The model under review builds one solid part; all positions refer to its coordinate system, in mm. Coordinates: 2 decimals unless noted, no trailing zeros. Order: outer loops, then holes, each group sorted by start corner. A loop starts at its lowest first (then second) coordinate and runs counter-clockwise, first axis right, second up.
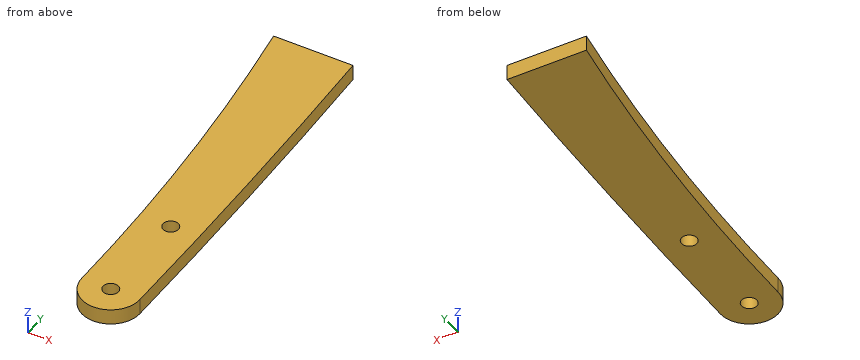
```python
from build123d import *

# Parameters (mm, degrees)
LEG_DEPTH       = 3.048
SKETCH4_R       = 1.524
FEETHOLES_DEPTH = 3.048


with BuildPart() as part:
    # Sketch3 → Leg (new body)
    with BuildSketch(Plane.XY):
        with BuildLine():
            Line((-11.667509286, 73.310783577), (3.98378723, 73.310783577))
            ThreePointArc((3.98378723, 73.310783577), (5.282136486, 36.665610885), (5.715, 0))
            ThreePointArc((5.715, 0), (0, -5.715), (-5.715, 0))
            ThreePointArc((-5.715, 0), (-7.20557197, 36.776022608), (-11.667509286, 73.310783577))
        make_face()
    extrude(amount=LEG_DEPTH)

    # Sketch4 → FeetHoles (cut)
    with BuildSketch(Plane.XY.offset(3.048)):
        Circle(SKETCH4_R)
        with Locations((0, 19.812)):
            Circle(SKETCH4_R)
    extrude(amount=-FEETHOLES_DEPTH, mode=Mode.SUBTRACT)


solid = part.part
```
(1) Wall thickness on probe 1 along Y at (x, z) = (0, 2.35) (3 decimals); probe 2 along Y at (x, z) = (1, 0.7); probe 3 along X at (y, z) = (49, 1.15): over which ranges is each line inside the solid? List them lowest first.
A:
probe 1: y = -5.715 to -1.524, 1.524 to 18.288, 21.336 to 73.311
probe 2: y = -5.63 to -1.15, 1.15 to 18.66, 20.96 to 73.31
probe 3: x = -8.36 to 4.94
(2) For pin 1 Ø2.5 at (x, y) = (0, 19.812) entering from +Z; pin 2 Ø1.5 at (y, z) = (13.5, 2) entering from -X, all flat-tipped, find the tip position at first contact; note any pin that passes through.
A:
pin 1: passes through
pin 2: stops at x = -5.94
(3) We need section D-D, the plane x = -10.5. Write out the cut boundary in (y, z).
A:
outline: (65.77, 0) - (73.31, 0) - (73.31, 3.05) - (65.77, 3.05) - close
(4) We need section B-B, the plane z = 0.7. Write out the cut boundary in (x, y) (1 decimal), and give its area (3 significant figures).
A:
outline: (-11.7, 73.3) arc R454.4 cw to (-5.7, 0) arc R5.7 ccw to (5.7, 0) arc R1553.1 ccw to (4, 73.3) - close; hole circle Ø3 at (0, 0); hole circle Ø3 at (0, 19.8)
area: 977 mm2
(5) We need section C-C, the plane y = 48.5. Write out the cut boundary in (x, z), and give its area (3 significant figures).
A:
outline: (-8.31, 0) - (4.96, 0) - (4.96, 3.05) - (-8.31, 3.05) - close
area: 40.4 mm2
(6) We need section A-A, the plane x = 0. Write out the cut boundary in (y, z) (3 decimals).
A:
outline: (-5.715, 0) - (-1.524, 0) - (-1.524, 3.048) - (-5.715, 3.048) - close; (1.524, 0) - (18.288, 0) - (18.288, 3.048) - (1.524, 3.048) - close; (21.336, 0) - (73.311, 0) - (73.311, 3.048) - (21.336, 3.048) - close
